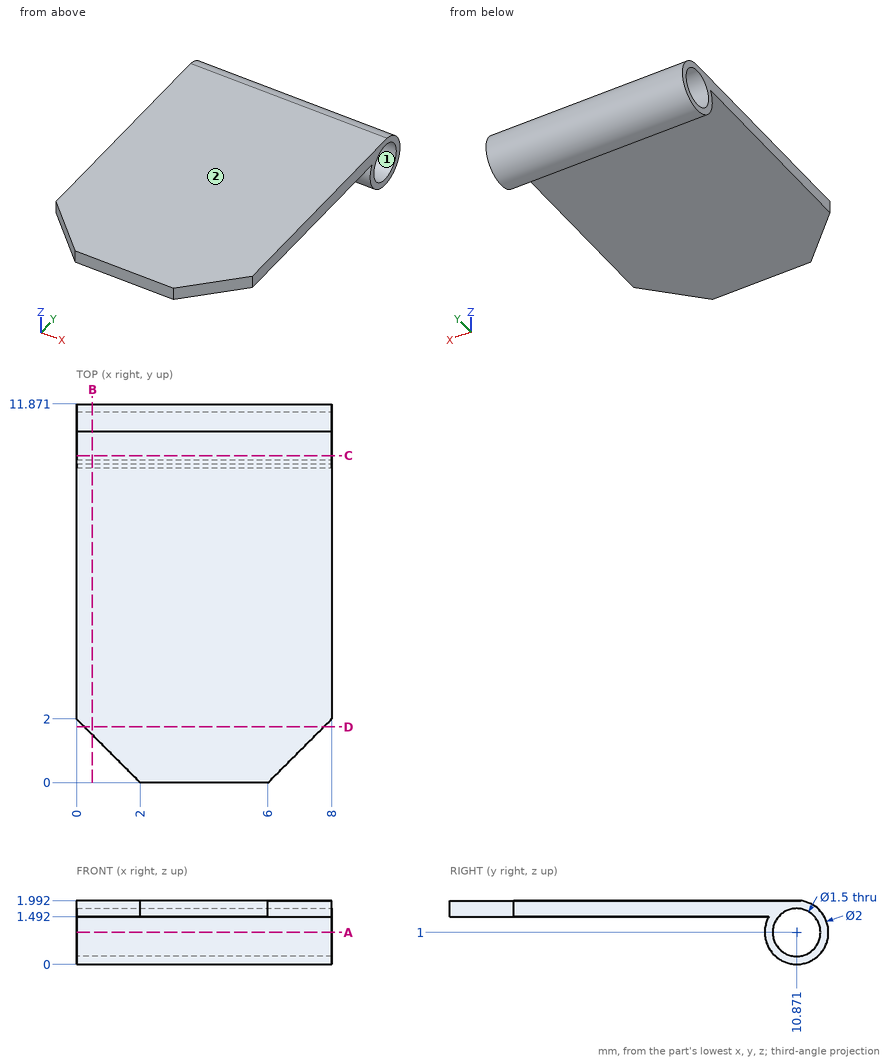
For this review, use the dimensioned drawing (mm, ordinates from the lowest corner) and the shaded views. Coordinates: 2 decimals unless noted, no trailing zeros. Loops run counter-clockwise (first coordinate to the right, second up) from the corner with the lowest first, then second, coordinate; pieces in that order, holes last.
1. Add section A-A, the plane z = 1. Give the boundary of the cut face in (x, y).
2. Insertion check: P1, Ø1, axis at x = 5.5, y = 7.5, coming from the -Z side. The pin has a flat end and moves straight along its axis. Give the tip position at first contact, or say it passes through.
3. Add section D-D, the plane y = 1.75. Give the boundary of the cut face in (x, z).
4. Add section C-C, the plane y = 10.25. Give the boundary of the cut face in (x, z).
5. Add section B-B, the plane x = 0.5. Give the boundary of the cut face in (y, z).
6. For line 1 (Z direction, x = 1, y = 2.5); line 2 (Z direction, x = 0.5, y = 10.25) (1 decimal); line 3 (Z direction, x = 1.75, y = 11), list the stretches that pass through material, from the lowest coordinate up.
7. Mouldability with a two-part tool opening along Z and no side actions: class the marked faces 1 and 2 as +Z half, -Z half, draft (parallel to the pull), parting line (faces both ways), or undercut.
Result:
1. outline: (0, 9.87) - (8, 9.87) - (8, 10.12) - (0, 10.12) - close; (0, 11.62) - (8, 11.62) - (8, 11.87) - (0, 11.87) - close
2. P1: stops at z = 1.49
3. outline: (0.25, 1.49) - (7.75, 1.49) - (7.75, 1.99) - (0.25, 1.99) - close
4. outline: (0, 0.22) - (8, 0.22) - (8, 0.58) - (0, 0.58) - close; (0, 1.42) - (8, 1.42) - (8, 1.99) - (0, 1.99) - close
5. outline: (1.5, 1.49) - (10, 1.49) arc R1 ccw (long way) to (11, 1.99) - (1.5, 1.99) - close; hole circle Ø1.5 at (10.87, 1)
6. line 1: z = 1.49 to 1.99
6. line 2: z = 0.2 to 0.6, 1.4 to 2
6. line 3: z = 0.01 to 0.26, 1.74 to 1.99
7. face 1: undercut
7. face 2: +Z half
